Part model, mm, in its own coordinate system. Face numbers are marked on the shaded views. Round coordinates to 2 decimals unless told otherwise and drop trailing zeros. Loops run counter-clockwise (first coordinate to the right, second up) from the corner with the lowest first, then second, coordinate; pieces in that order, holes last. Notation, with made-up numbers: (64.25, 84.25) -> (99.25, 84.25) arc R8 cw to (99.25, 91.25) -> close; hole circle Ø7 at (79.5, 28). An arc over 180 degrees is marked (long way). Answer as CSV lines item,"result".
from build123d import *

# Parameters (mm, degrees)
F0_W     = 20
F0_H     = 20
F0_R     = 3.5
F1_DEPTH = 7
F2_R     = 2
F3_R     = 1.5
F4_DEPTH = 25


with BuildPart() as f1:
    # F0 (on Top) → F1 (new body)
    with BuildSketch(Plane.XY):
        Rectangle(F0_W, F0_H)
        Circle(F0_R, mode=Mode.SUBTRACT)
    extrude(amount=F1_DEPTH)

    # F2
    f2_edges = [f1.edges().sort_by_distance(p)[0] for p in [
        (0, -10, 7),
        (0, -10, 0),
        (0, 10, 7),
        (0, 10, 0),
    ]]
    fillet(f2_edges, radius=F2_R)

    # F3 (on face) → F4 (cut)
    with BuildSketch(Plane(origin=(-10, 0, 0), x_dir=(0, -1, 0), z_dir=(-1, 0, 0))):
        with Locations((-6, 3.5)):
            Circle(F3_R)
        with Locations((6, 3.5)):
            Circle(F3_R)
    extrude(amount=-F4_DEPTH, mode=Mode.SUBTRACT)


solid = f1.part
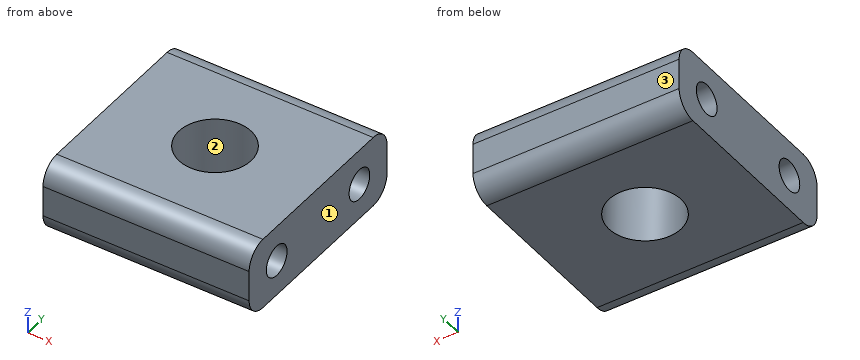
Q1. Saw through at B-B, the plane x = -5.25. Write the cut outline in (y, z), then the cut area to 3 significant figures.
Geometry results:
outline,"(-10, 2) arc R2 ccw to (-8, 0) -> (8, 0) arc R2 ccw to (10, 2) -> (10, 5) arc R2 ccw to (8, 7) -> (-8, 7) arc R2 ccw to (-10, 5) -> close; hole circle Ø3 at (-6, 3.5); hole circle Ø3 at (6, 3.5)"
area,"122 mm2"
Q2. Saw through at C-C, the plane y = 6. Write the cut outline in (x, z).
Geometry results:
outline,"(-10, 0) -> (10, 0) -> (10, 2) -> (-10, 2) -> close; (-10, 5) -> (10, 5) -> (10, 7) -> (-10, 7) -> close"
Q3. Saw through at A-A, the plane z = 3.5. Write the cut outline in (x, y).
Geometry results:
outline,"(-10, -10) -> (10, -10) -> (10, -7.5) -> (-10, -7.5) -> close; (-10, -4.5) -> (10, -4.5) -> (10, 4.5) -> (-10, 4.5) -> close; (-10, 7.5) -> (10, 7.5) -> (10, 10) -> (-10, 10) -> close; hole circle Ø7 at (0, 0)"
Q4. Two-plate mould, pull along X, no slides. Class the marked faces 1, 2 and 3: pulls with the +X half, pulls with the -X half, needs draft (parallel to the pull), parting line crosses it, or undercut.
Geometry results:
face 1,"pulls with the +X half"
face 2,"undercut"
face 3,"needs draft"
Q5. Saw through at D-D, the plane x = -1. Write the cut outline in (y, z).
Geometry results:
outline,"(-10, 2) arc R2 ccw to (-8, 0) -> (-3.35, 0) -> (-3.35, 7) -> (-8, 7) arc R2 ccw to (-10, 5) -> close; (3.35, 0) -> (8, 0) arc R2 ccw to (10, 2) -> (10, 5) arc R2 ccw to (8, 7) -> (3.35, 7) -> close; hole circle Ø3 at (-6, 3.5); hole circle Ø3 at (6, 3.5)"
Q6. Drill centre lines: line 1 along Y through (x, z) = (-9, 4.5); line 2 along Z through (x, y) = (-4.5, -6); line 3 along X through (y, z) = (1, 6.5). Where is each one in solid material? Low to high.
Geometry results:
line 1,"-10 to -7.12, -4.88 to 4.88, 7.12 to 10"
line 2,"0 to 2, 5 to 7"
line 3,"-10 to -3.35, 3.35 to 10"
Q7. Drop a flat-ended pin along its axis: P1, Ø6.5, axis at x = 0, y = 0, coming from the -Z side. Give the stop position or say it passes through.
Geometry results:
P1,"through"
